Could you check a few things on this drawing? It's one solid part, dimensions in mm from its lowest x, y, z. A direction names the side the tool comes from. Round coordinates to 2 decimals unless told otherwise and drop trailing zeros. Write each loop counter-clockwise with the first axis right and the second up, starting at its lowest first coordinate (ties: lowest second). Pieces come first, ordered by that corner, then holes. Notation, with made-up numbers: (-3.75, 88) -> (9.25, 88) arc R8 cw to (9.25, 98) -> close; hole circle Ø10 at (71.25, 6). An arc over 180 degrees is marked (long way). Put each result on its own line as item: value. Start each with the question number.
1) Which directions (+Z, -Z, +X, -X, +Y, -Y) give clear straight access to the entire face, cutting with the end or side of a thin tool? Please do the marked faces 4, 5 and 6.
2) We'd pull the mould along Z, two halves only. Please class the marked faces 1, 2 and 3: released by +Z, released by -Z, zero draft, split by the parting line, or undercut.
3) I want a section at A-A, the plane x = 37.25. List the corners of the cut face in (y, z) for me.
4) I want a section at D-D, the plane x = 19.5. List the corners of the cut face in (y, z) for me.
5) If I drill on line 1 along X through (y, z) = (13.5, 37.5); line 2 along X through (y, z) = (16.75, 75); line 3 along Y through (x, z) = (23, 66), over which ranges is the centre line in solid material (lowest first)? Write a range as [from, to].
6) I want a section at C-C, the plane y = 18. Give the number of separate pieces and of enclosed holes in the cut face.
7) Will these pins go through, and if not, where does the flat tip stop? P1, Ø8, axis at x = 8, z = 38.5, coming from the +Y side; P2, Ø12.5, axis at y = 18, z = 71, coming from the +X side (1 decimal); P3, Ø6, axis at y = 18, z = 79.63, coming from the +X side; P4, Ø3.5, axis at x = 48.08, z = 43.5, coming from the +Y side.
8) I want a section at B-B, the plane z = 37.25. List the corners of the cut face in (x, y) for me.
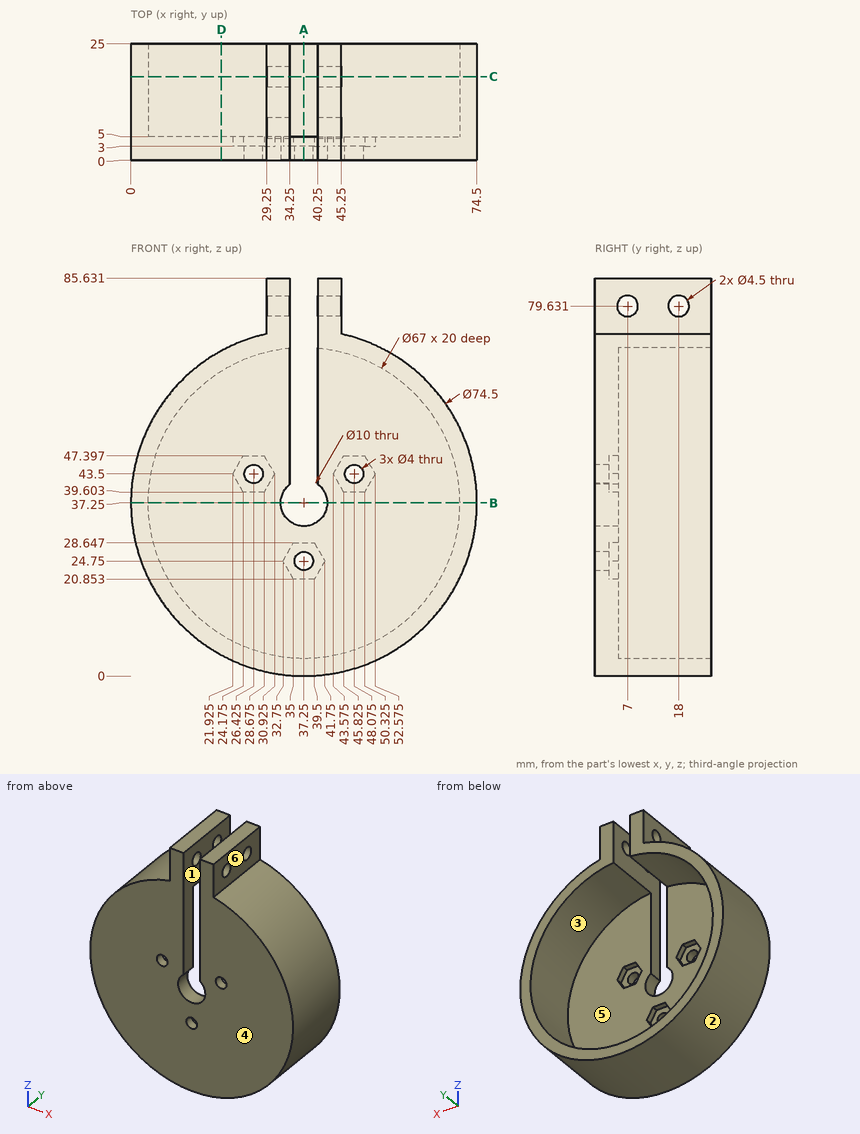
Findings:
1. face 4: +Z, -Z, +X, -X, -Y
1. face 5: +Y
1. face 6: +Z, +X, +Y, -Y
2. face 1: zero draft
2. face 2: split by the parting line
2. face 3: undercut
3. outline: (0, 0) -> (25, 0) -> (25, 3.75) -> (5, 3.75) -> (5, 20.85) -> (3, 20.85) -> (3, 22.75) -> (0, 22.75) -> close; (0, 26.75) -> (3, 26.75) -> (3, 28.65) -> (5, 28.65) -> (5, 32.25) -> (0, 32.25) -> close
4. outline: (0, 4.5) -> (25, 4.5) -> (25, 8.84) -> (5, 8.84) -> (5, 65.66) -> (25, 65.66) -> (25, 70) -> (0, 70) -> close
5. line 1: x = [0, 3.75], [70.75, 74.5]
5. line 2: x = [29.25, 34.25], [40.25, 45.25]
5. line 3: y = [0, 5]
6. separate pieces: 3
6. enclosed holes: 0
7. P1: stops at y = 5
7. P2: stops at x = 62.4
7. P3: stops at x = 45.25
7. P4: passes through
8. outline: (0, 0) -> (32.25, 0) -> (32.25, 5) -> (3.75, 5) -> (3.75, 25) -> (0, 25) -> close; (42.25, 0) -> (74.5, 0) -> (74.5, 25) -> (70.75, 25) -> (70.75, 5) -> (42.25, 5) -> close
